Here's the drawing with two shaded views (mm, measured from the low corner). I have some questions. A direction names the side the tool comes from. Round coordinates to 2 decimals unless told otherwise and drop trailing zeros. Return JSON: item names as keys, results as strings. Group by question number.
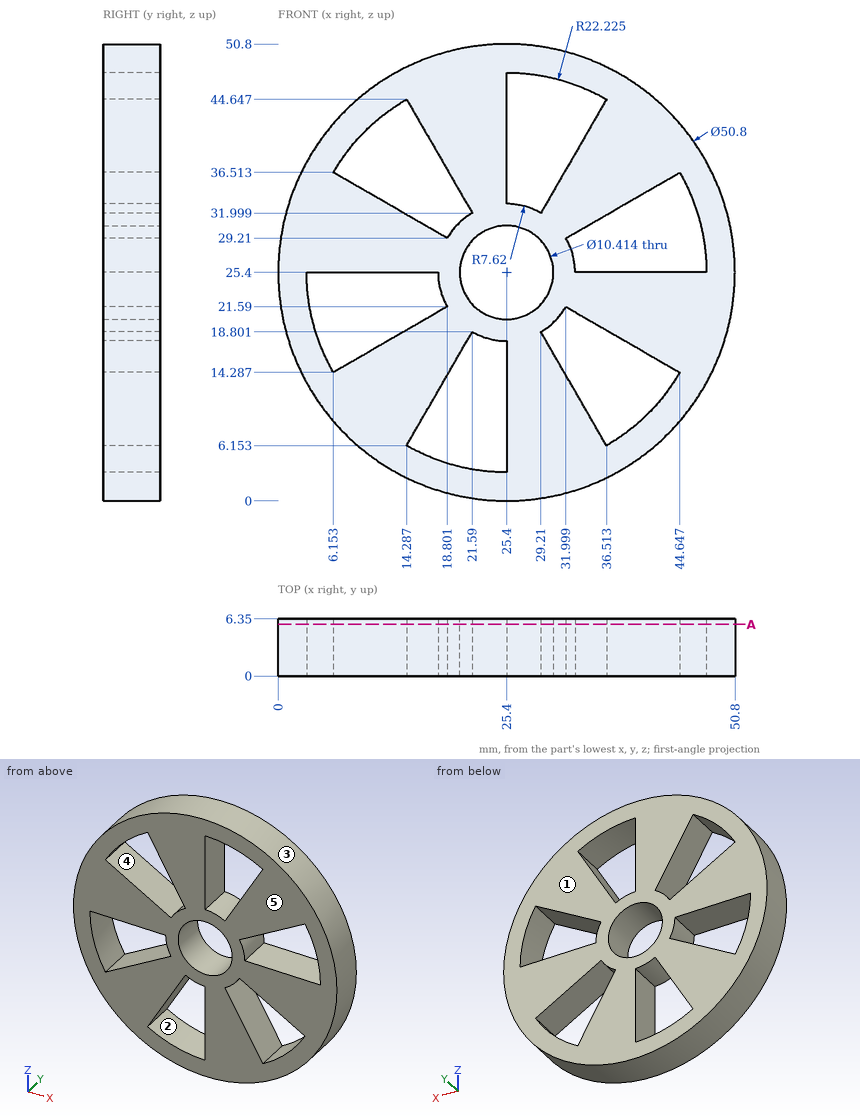
1) If I drill on line 1 along X through (y, z) = (0.5, 22) (1 decimal); line 2 along X through (y, z) = (3.5, 41.5) (1 decimal); line 3 along Z through (x, y) = (28, 2.5) (1 decimal), over which ranges is the centre line in solid material (lowest first)? Write a range as from..to.
2) For the marked faces 1 and 2, which set-ups out of +Z, -Z, +X, -X, +Y, -Y let a thin tool reach every point of the face, with its end or its side?
3) We'd pull the mould along Z, two halves only. Please class the marked faces 3, 4 and 5: +Z half, -Z half, draft (parallel to the pull), parting line (faces both ways), or undercut.
4) Will these pins go through, and if not, where does the flat tip stop? pin 1 (1.5 mm diameter, centred on y = 4.5, z = 31.5, fed in from -X); pin 2 (2 mm diameter, centred on x = 24.5, z = 37, fed in from -Y); pin 3 (3 mm diameter, centred on x = 39, y = 2.5, fed in from -Z); pin 4 (2 mm diameter, centred on y = 5, z = 41, fed in from +X) (1 decimal).
5) I want a section at A-A, the plane y = 5.75. Give the number of separate pieces and of enclosed holes in the cut face, plus the area to 3 significant figures.
Outcome:
{
 "1": {"line 1": "0.2..3.4, 18.6..21.5, 29.3..50.6", "line 2": "5.8..10.1, 16.1..25.4, 34.7..45", "line 3": "0.1..20.9, 29.9..32.6, 47.5..50.7"},
 "2": {"face 1": "+Z, -Z, +X, -X, +Y", "face 2": "+Y, -Y"},
 "3": {"face 3": "parting line", "face 4": "undercut", "face 5": "draft"},
 "4": {"pin 1": "x = 0.57", "pin 2": "y = 0", "pin 3": "z = 3.07", "pin 4": "x = 46.2"},
 "5": {"separate pieces": "1", "enclosed holes": "7", "area": "1,260 mm^2"}
}
